```python
from build123d import *

# Parameters (mm, degrees)
F0_R      = 8
F1_DEPTH  = 12
F3_DEPTH  = 126
F4_R      = 34
F5_DEPTH  = 26
F6_DEPTH  = 40
F7_R      = 15
F8_DEPTH  = 66
F10_DEPTH = 14


with BuildPart() as f1:
    # F0 (on Top) → F1 (new body)
    with BuildSketch(Plane.XY):
        with BuildLine():
            ThreePointArc((-60, -66), (-55.313708, -77.313708), (-44, -82))
            Line((-44, -82), (44, -82))
            ThreePointArc((44, -82), (55.313708, -77.313708), (60, -66))
            Line((60, -66), (60, 44))
            ThreePointArc((60, 44), (55.313708, 55.313708), (44, 60))
            Line((44, 60), (0, 60))
            Line((0, 60), (-44, 60))
            ThreePointArc((-44, 60), (-55.313708, 55.313708), (-60, 44))
            Line((-60, 44), (-60, -66))
        make_face()
        with Locations((-44, -66)):
            Circle(F0_R, mode=Mode.SUBTRACT)
        with Locations((44, -66)):
            Circle(F0_R, mode=Mode.SUBTRACT)
        with Locations((-44, 44)):
            Circle(F0_R, mode=Mode.SUBTRACT)
        with Locations((44, 44)):
            Circle(F0_R, mode=Mode.SUBTRACT)
    extrude(amount=F1_DEPTH)

    # F2 (on face) → F3 (join)
    with BuildSketch(Plane.XY.offset(12)):
        Polygon((7, 60), (0, 60), (-7, 60), (-7, -66), (7, -66), align=None)
    extrude(amount=F3_DEPTH)

    # F4 (on face) → F5 (join)
    with BuildSketch(Plane(origin=(-7, 0, 0), x_dir=(0, -1, 0), z_dir=(-1, 0, 0))):
        with Locations((46, 138)):
            Circle(F4_R)
    extrude(amount=F5_DEPTH)

    # F4 (on face) → F6 (join)
    with BuildSketch(Plane(origin=(-7, 0, 0), x_dir=(0, -1, 0), z_dir=(-1, 0, 0))):
        with Locations((46, 138)):
            Circle(F4_R)
    extrude(amount=-F6_DEPTH)

    # F7 (on face) → F8 (cut)
    with BuildSketch(Plane(origin=(-33, 0, 0), x_dir=(0, -1, 0), z_dir=(-1, 0, 0))):
        with Locations((46, 138)):
            Circle(F7_R)
    extrude(amount=-F8_DEPTH, mode=Mode.SUBTRACT)

    # F9 (on face) → F10 (cut)
    with BuildSketch(Plane(origin=(-7, 0, 0), x_dir=(0, -1, 0), z_dir=(-1, 0, 0))):
        Polygon((-60, 12), (12, 138), (-60, 138), align=None)
    extrude(amount=-F10_DEPTH, mode=Mode.SUBTRACT)


solid = f1.part
```
Geometry check sheet. Reference: the model listing, model coordinates, mm. A direction names the side the tool comes from. Coordinates: 2 decimals unless noted, no trailing zeros. Order: outer loops, then holes, each group sorted by start corner. A loop starts at its lowest first (then second) coordinate and runs counter-clockwise, first axis right, second up.
Item 1: Section check A-A (x = -27). Enter the section's corners in (y, z), plus the area to 3 significant figures.
Item 2: Depth check by flat-ended pin: pin 1 (18.5 mm diameter, centred on x = 44, y = 44, fed in from +Z); pin 2 (8 mm diameter, centred on x = -32, z = 142.5, fed in from -Y); pin 3 (14.5 mm diameter, centred on x = -44, y = 44, fed in from -Z); pin 4 (4 mm diameter, centred on x = -1.5, z = 84, fed in from -Y). Enter the tip coordinate at first touch or a pass-through.
Item 3: Tool access check on faces 4 (the cylindrical face through (-45.041, -58.068, 5.916)), 5 (the flat face through (33, -61, 131)), 6 (the flat face through (0, -66, 61)). Record the directions out of +Z, -Z, +X, -X, +Y, -Y that give a thin tool (end or side, any length) a straight path to the whole face; none if there is none.
Item 4: Mould release check, pull along Y, two halves, no side actions. Record for faces 1 (the flat face through (-7, -16, 60)), 2 (the cylindrical face through (42.959, -58.068, 5.916)), 3 (the flat face through (1, 60, 6)): released by +Y, released by -Y, zero draft, split by the parting line, or undercut.
Item 5: Section check B-B (y = -46). Enter the section's corners in (x, z).
Item 6: Section check D-D (y = -28). Enter the section's corners in (x, z).
Item 7: Section check C-C (z = 126). Enter the section's corners in (x, y), plus the area to 3 significant figures.
Item 8: Scan lines: line 1 along Y through (x, z) = (-44, 3); line 2 along Z through (x, y) = (12.5, 25); line 3 along X through (y, z) = (-54, 92). Record each from-to range of solid material in increasing order.
Check sheet entries:
1. outline: (-82, 0) - (60, 0) - (60, 12) - (-82, 12) - close; circle Ø68 at (-46, 138); hole circle Ø30 at (-46, 138)
1. area: 4,630 mm2
2. pin 1: stops at z = 12
2. pin 2: stops at y = -80
2. pin 3: passes through
2. pin 4: stops at y = -66
3. face 4: +Z, -Z
3. face 5: +Z, +X, +Y, -Y
3. face 6: +X, -X, -Y
4. face 1: zero draft
4. face 2: undercut
4. face 3: released by +Y
5. outline: (-60, 0) - (60, 0) - (60, 12) - (7, 12) - (7, 104) - (33, 104) - (33, 123) - (-33, 123) - (-33, 104) - (-7, 104) - (-7, 12) - (-60, 12) - close; (-33, 153) - (33, 153) - (33, 172) - (-33, 172) - close
6. outline: (-60, 0) - (60, 0) - (60, 12) - (7, 12) - (7, 109.16) - (33, 109.16) - (33, 166.84) - (-33, 166.84) - (-33, 109.16) - (-7, 109.16) - (-7, 12) - (-60, 12) - close
7. outline: (-33, -77.81) - (33, -77.81) - (33, -55) - (-33, -55) - close; (-33, -37) - (33, -37) - (33, -14.19) - (7, -14.19) - (7, -5.14) - (-7, -5.14) - (-7, -14.19) - (-33, -14.19) - close
7. area: 3,140 mm2
8. line 1: y = -82 to -74, -58 to 36, 52 to 60
8. line 2: z = 0 to 12
8. line 3: x = -7 to 7
